Study the drawing (mm; zero at the part's minimum x, y, z) and answer. Round coordinates to 2 decimals unless told otherwise and drop trailing zeros. Write each loop counter-clockwise with the first axis right and the second up, starting at its lowest first coordinate (ties: lowest second). Pieces come first, ordered by that corner, then holes. Notation, with made-up numbers: (-2.75, 78) -> (17.25, 78) arc R24 ccw to (17.25, 95) -> close; hole circle Ø10 at (6, 21). An arc over 180 degrees is marked (long way). Return JSON: item names as keys, results as strings.
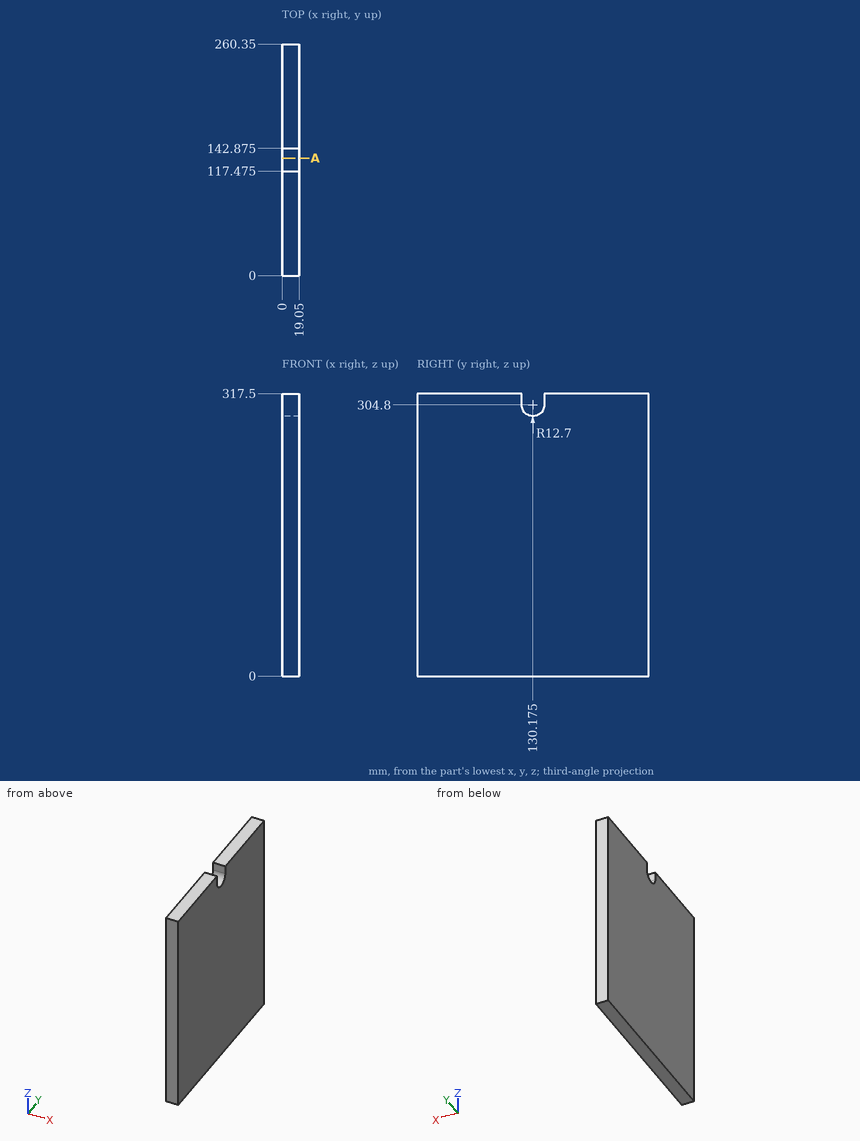
Item 1: Straight lines are drawn through the part: L1, parallel to Y at x = 2.5, z = 300.5; L2, parallel to Z at x = 14, y = 120. For each, find the intervals that lie inside material, in ascending order. Write a range as [from, to].
Worked answers:
{"L1": "y = [0, 118.23], [142.12, 260.35]", "L2": "z = [0, 297.2]"}
Item 2: Section A-A (y = 132) is taken. Give the vertices of the cut face in (x, z), then the cut area to 3 significant figures.
Worked answers:
{"outline": "(0, 0) -> (19.05, 0) -> (19.05, 292.23) -> (0, 292.23) -> close", "area": "5,570 mm2"}
Item 3: A flat-ended cylindrical pin translates along its axis: pin 1 (2 mm diameter, centred on y = 130, z = 164.5, fed in from -X). Find the tip coordinate at first contact, or state that the pin passes through.
Worked answers:
{"pin 1": "stops at x = 0"}
